Source: three-view drawing plus pictorial views. Frame: mm from the lowest corner of the part. A direction names the side the tool comes from. Round coordinates to 2 decimals unless told otherwise and drop trailing zeros. Loops run counter-clockwise (first coordinate to the right, second up) from the corner with the lowest first, then second, coordinate; pieces in that order, holes last. Notation, with made-up numbers: (46.25, 14.25) -> (74.25, 14.25) arc R15 cw to (74.25, 31.25) -> close; hole circle Ø10 at (82, 44.5). An arc over 180 degrees is marked (long way). Put each result on its own line as item: value. Start each with the question number.
1. Material intervals for L1, parallel to X at y = 4.25, z = 12.5; L2, parallel to X at y = 9, z = 56; L3, parallel to Y at x = 16.5, z = 37, sorted ascending.
2. Contact query for flat-ended pins moving along their axis: pin 1 (25 mm diameter, centred on x = 17.5, z = 33.5, fed in from +Y); pin 2 (2.5 mm diameter, centred on y = 1.5, z = 16.5, fed in from +X); pin 3 (4 mm diameter, centred on x = 44.5, y = 4.5, fed in from +Z); pin 4 (5.5 mm diameter, centred on x = 13.5, y = 9, fed in from +Z). Output: stop coordinate, or through.
3. Set-up query: the marked faces 1, 2 and 3. Return all of +Z, -Z, +X, -X, +Y, -Y with unobstructed straight access to the full face (end or side cutting, diameter ignored); none if empty.
4. Cut plane C-C (x = 19.5). Return the cut outline in (y, z).
5. Cut plane D-D (z = 30.5). Return the cut outline in (x, y), then the cut area to 3 significant figures.
6. Cut plane A-A (y = 2.75). Return the cut outline in (x, z).
7. Cut plane B-B (y = 10.25). Return the cut outline in (x, z).
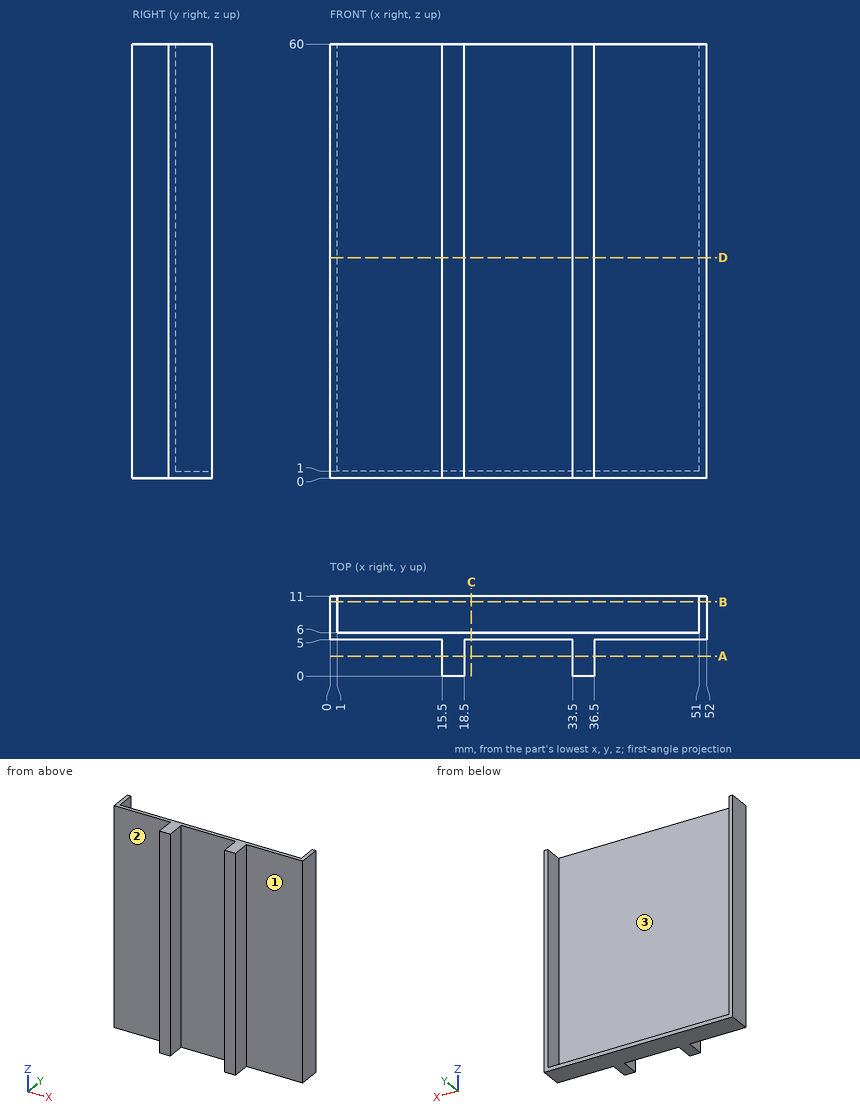
Solution:
1. L1: x = 15.5 to 18.5, 33.5 to 36.5
1. L2: x = 0 to 1, 51 to 52
1. L3: y = 0 to 6
2. pin 1: stops at y = 6
2. pin 2: stops at x = 36.5
2. pin 3: stops at z = 60
2. pin 4: stops at z = 1
3. face 1: +Z, -Z, +X, -Y
3. face 2: +Z, -Z, -X, -Y
3. face 3: +Z, +Y
4. outline: (5, 0) -> (11, 0) -> (11, 1) -> (6, 1) -> (6, 60) -> (5, 60) -> close
5. outline: (0, 5) -> (15.5, 5) -> (15.5, 0) -> (18.5, 0) -> (18.5, 5) -> (33.5, 5) -> (33.5, 0) -> (36.5, 0) -> (36.5, 5) -> (52, 5) -> (52, 11) -> (51, 11) -> (51, 6) -> (1, 6) -> (1, 11) -> (0, 11) -> close
5. area: 92.0 mm^2
6. outline: (15.5, 0) -> (18.5, 0) -> (18.5, 60) -> (15.5, 60) -> close; (33.5, 0) -> (36.5, 0) -> (36.5, 60) -> (33.5, 60) -> close
7. outline: (0, 0) -> (52, 0) -> (52, 60) -> (51, 60) -> (51, 1) -> (1, 1) -> (1, 60) -> (0, 60) -> close
